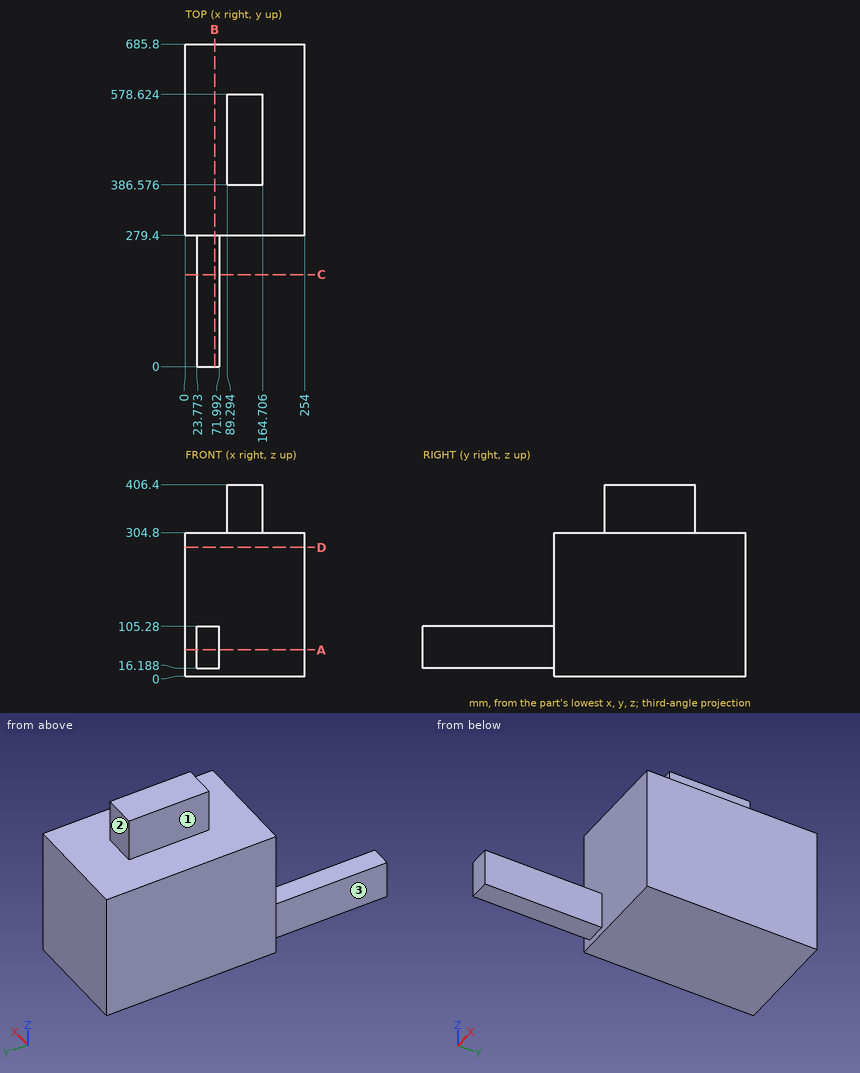
Could you check a few things on this drawing? It's one solid part, dimensions in mm from its lowest x, y, z. A direction names the side the tool comes from. Round coordinates to 2 decimals unless told otherwise and drop trailing zeros. Write each loop counter-clockwise with the first axis right and the second up, starting at its lowest first coordinate (ties: lowest second). Pieces come first, ordered by that corner, then holes. Notation, with made-up numbers: (51, -11) -> (64, -11) arc R17 ccw to (64, 8) -> close; hole circle Ø4 at (35, -25). An arc over 180 degrees is marked (long way). One line per item, written item: value.
1) Suppose I cut it at C-C on y = 195.5. List the corners of the cut face in (x, z) for me.
Filled sheet:
outline: (23.77, 16.19) -> (71.99, 16.19) -> (71.99, 105.28) -> (23.77, 105.28) -> close
2) Suppose I cut it at A-A on z = 55.5. List the corners of the cut face in (x, y) for me, plus the area to 3 significant figures.
Filled sheet:
outline: (0, 279.4) -> (23.77, 279.4) -> (23.77, 0) -> (71.99, 0) -> (71.99, 279.4) -> (254, 279.4) -> (254, 685.8) -> (0, 685.8) -> close
area: 117,000 mm2
3) Suppose I cut it at B-B on x = 62. List the corners of the cut face in (y, z) for me, plus the area to 3 significant figures.
Filled sheet:
outline: (0, 16.19) -> (279.4, 16.19) -> (279.4, 0) -> (685.8, 0) -> (685.8, 304.8) -> (279.4, 304.8) -> (279.4, 105.28) -> (0, 105.28) -> close
area: 149,000 mm2
4) If I drill on line 1 (Y direction, x = 92.5, z = 83.5); line 2 (Z direction, x = 68, y = 357); line 3 (Y direction, x = 111, z = 336), over which ranges is the centre line in solid material (lowest first)? Write a range as [from, to].
Filled sheet:
line 1: y = [279.4, 685.8]
line 2: z = [0, 304.8]
line 3: y = [386.58, 578.62]
5) I'm going to push flat-ended pins straight in: pin 1 Ø6 at (x, y) = (66, 158.5) entering from -Z; pin 2 Ø1.5 at (x, y) = (37.5, 413) entering from +Z; pin 3 Ø22.5 at (x, z) = (135, 344) entering from -Y. Where does each tip first touch, or does it pass through?
Filled sheet:
pin 1: stops at z = 16.19
pin 2: stops at z = 304.8
pin 3: stops at y = 386.58
6) Suppose I cut it at D-D on z = 273.5. List the corners of the cut face in (x, y) for me, plus the area to 3 significant figures.
Filled sheet:
outline: (0, 279.4) -> (254, 279.4) -> (254, 685.8) -> (0, 685.8) -> close
area: 103,000 mm2
7) For the marked faces 1, 2 and 3, which set-ups out of +Z, -Z, +X, -X, +Y, -Y let a thin tool reach every point of the face, with its end or its side?
Filled sheet:
face 1: +Z, -X, +Y, -Y
face 2: +Z, +X, -X, +Y
face 3: +Z, -Z, -X, -Y
